from build123d import *

# Parameters (mm, degrees)
BOSS_EXTRUDE1_DEPTH = 3.175
SKETCH1_4_R         = 3.125
CUT_EXTRUDE1_DEPTH  = 439.905857431
FILLET1_R           = 48
CUT_EXTRUDE3_DEPTH  = 10
CUT_EXTRUDE5_REACH  = 440.906
SKETCH12_R          = 4.625


with BuildPart() as part:
    # Sketch1 → Boss-Extrude1 (new body)
    with BuildSketch(Plane.XY):
        Polygon((-98.879411765, 3.850980392), (-31.879411765, -96.649019608), (366, -96.649019608), (403.120588235, -71.149019608), (428.120588235, 28.939617947), (-115.605170134, 28.939617947), align=None)
    extrude(amount=BOSS_EXTRUDE1_DEPTH)

    # Sketch1<4> → Cut-Extrude1 (cut, through all)
    with BuildSketch(Plane.XY):
        with Locations((-12.879411765, -83.899019608)):
            Circle(SKETCH1_4_R)
        with Locations((51.120588235, -83.899019608)):
            Circle(SKETCH1_4_R)
        with Locations((115.120588235, -83.899019608)):
            Circle(SKETCH1_4_R)
        with Locations((179.120588235, -83.899019608)):
            Circle(SKETCH1_4_R)
        with Locations((243.120588235, -83.899019608)):
            Circle(SKETCH1_4_R)
        with Locations((307.120588235, -83.899019608)):
            Circle(SKETCH1_4_R)
    extrude(amount=CUT_EXTRUDE1_DEPTH, mode=Mode.SUBTRACT)

    # Fillet1
    fillet1_edges = [part.edges().sort_by_distance(p)[0] for p in [
        (-31.879411765, -96.649019608, 1.5875),
    ]]
    fillet(fillet1_edges, radius=FILLET1_R)

    # Sketch7 → Cut-Extrude3 (cut)
    with BuildSketch(Plane.XY.offset(3.175)):
        Polygon((403.120588235, -71.149019608), (340.005873473, -96.649019608), (366, -96.649019608), align=None)
    extrude(amount=-CUT_EXTRUDE3_DEPTH, mode=Mode.SUBTRACT)

    # Sketch12 → Cut-Extrude5 (cut, up to next)
    with BuildSketch(Plane.XY.offset(3.175), mode=Mode.PRIVATE) as cut_extrude5_sk1:
        with Locations((397.677759779, -24.610405856)):
            Circle(SKETCH12_R)
    cut_extrude5_tool1 = extrude(cut_extrude5_sk1.sketch, amount=-CUT_EXTRUDE5_REACH, mode=Mode.PRIVATE) & part.part
    add(cut_extrude5_tool1.solids().sort_by_distance((397.67776, -24.610406, 3.175))[0], mode=Mode.SUBTRACT)


solid = part.part
Input: part model. Units: mm. Frame: model coordinates. Round coordinates to 2 decimals unless told otherwise and drop trailing zeros. Write each loop counter-clockwise with the first axis right and the second up, starting at its lowest first coordinate (ties: lowest second). Pieces come first, ordered by that corner, then holes.
1) Cut plane B-B (x = -22). Return the cut outline in (y, z) (3 decimals), then the cut area to 3 significant figures.
2) Cut plane A-A (z = 1.25). Return the cut outline in (x, y) (3 decimals), then the cut area to 3 significant figures.
3) Cut plane C-C (y = -65.5). Return the cut outline in (x, z) (3 decimals).
4) Ray query, L1, parallel to Y at x = 309, z = 3; L2, parallel to X at y = -56, z = 1.8; L3, parallel to Y at x = -83.5, z = 2.75. Return the intervals inside material, ascending.
5) Draft query along Y for faces 1 (the flat face through (152, -33, 0)), 2 (the cylindrical face through (393.057, -24.407, 1.61)), 3 (the flat face through (415.446, -21.805, 1.565)). Return one class per face: pulls with the +Y half, pulls with the -Y half, needs draft (parallel to the pull), parting line crosses it, or undercut.
Geometry says:
1. outline: (-93.971, 0) - (28.94, 0) - (28.94, 3.175) - (-93.971, 3.175) - close
1. area: 390 mm2
2. outline: (-115.605, 28.94) - (-46.129, -75.275) arc R48 ccw to (-6.191, -96.649) - (340.006, -96.649) - (403.121, -71.149) - (428.121, 28.94) - close; hole circle Ø6.25 at (-12.879, -83.899); hole circle Ø6.25 at (51.121, -83.899); hole circle Ø6.25 at (115.121, -83.899); hole circle Ø6.25 at (179.121, -83.899); hole circle Ø6.25 at (243.121, -83.899); hole circle Ø6.25 at (307.121, -83.899); hole circle Ø9.25 at (397.678, -24.61)
2. area: 60,000 mm2
3. outline: (-52.645, 0) - (404.532, 0) - (404.532, 3.175) - (-52.645, 3.175) - close
4. L1: y = -96.65 to -86.4, -81.4 to 28.94
4. L2: x = -58.98 to 406.9
4. L3: y = -19.22 to 28.94
5. face 1: needs draft
5. face 2: undercut
5. face 3: pulls with the -Y half
